from build123d import *

# Parameters (mm, degrees)
SKETCH1_R           = 1.6
SKETCH1_R_2         = 20
BOSS_EXTRUDE2_DEPTH = 1.7
BOSS_EXTRUDE3_START = -1.7
SKETCH2_R           = 1.5
BOSS_EXTRUDE3_DEPTH = 1.7
SKETCH3_W           = 67.365157796
SKETCH3_H           = 36
CUT_EXTRUDE1_DEPTH  = 1.7
FILLET1_R           = 3


with BuildPart() as part:
    # Sketch1 → Boss-Extrude2 (new body)
    with BuildSketch(Plane(origin=(0, 0, 0), x_dir=(1, 0, 0), z_dir=(0, 1, 0))):
        with BuildLine():
            Line((-17.673720383, -21.068687852), (-2.459890554, -40.906514899))
            ThreePointArc((-2.459890554, -40.906514899), (0, -42.12), (2.459890554, -40.906514899))
            Line((2.459890554, -40.906514899), (17.673720383, -21.068687852))
            ThreePointArc((17.673720383, -21.068687852), (19.445436483, -19.445436483), (21.068687852, -17.673720383))
            Line((21.068687852, -17.673720383), (40.906514899, -2.459890554))
            ThreePointArc((40.906514899, -2.459890554), (42.12, 0), (40.906514899, 2.459890554))
            Line((40.906514899, 2.459890554), (21.068687852, 17.673720383))
            ThreePointArc((21.068687852, 17.673720383), (19.445436483, 19.445436483), (17.673720383, 21.068687852))
            Line((17.673720383, 21.068687852), (2.459890554, 40.906514899))
            ThreePointArc((2.459890554, 40.906514899), (0, 42.12), (-2.459890554, 40.906514899))
            Line((-2.459890554, 40.906514899), (-17.673720383, 21.068687852))
            ThreePointArc((-17.673720383, 21.068687852), (-19.445436483, 19.445436483), (-21.068687852, 17.673720383))
            Line((-21.068687852, 17.673720383), (-40.906514899, 2.459890554))
            ThreePointArc((-40.906514899, 2.459890554), (-42.12, 0), (-40.906514899, -2.459890554))
            Line((-40.906514899, -2.459890554), (-21.068687852, -17.673720383))
            ThreePointArc((-21.068687852, -17.673720383), (-19.445436483, -19.445436483), (-17.673720383, -21.068687852))
        make_face()
        with Locations(Location((0, -39.02, 0), (0, 0, 270))):
            Circle(SKETCH1_R, mode=Mode.SUBTRACT)
        with Locations(Location((0, 0, 0), (0, 0, 270))):
            Circle(SKETCH1_R_2, mode=Mode.SUBTRACT)
        with Locations(Location((-39.02, 0, 0), (0, 0, 270))):
            Circle(SKETCH1_R, mode=Mode.SUBTRACT)
        with Locations(Location((39.02, 0, 0), (0, 0, 270))):
            Circle(SKETCH1_R, mode=Mode.SUBTRACT)
        with Locations(Location((0, 39.02, 0), (0, 0, 270))):
            Circle(SKETCH1_R, mode=Mode.SUBTRACT)
    extrude(amount=BOSS_EXTRUDE2_DEPTH)

    # Sketch2 → Boss-Extrude3 (add)
    with BuildSketch(Plane(origin=(0, 1.7, 0), x_dir=(1, 0, 0), z_dir=(0, 1, 0)).offset(BOSS_EXTRUDE3_START)):
        with BuildLine():
            Line((-30.78, -47.52), (-30.78, -10.226017059))
            Line((-30.78, -10.226017059), (-21.068687852, -17.673720383))
            ThreePointArc((-21.068687852, -17.673720383), (-19.445436483, -19.445436483), (-17.673720383, -21.068687852))
            Line((-17.673720383, -21.068687852), (-2.459890554, -40.906514899))
            ThreePointArc((-2.459890554, -40.906514899), (0, -42.12), (2.459890554, -40.906514899))
            ThreePointArc((2.459890554, -40.906514899), (-3.472049402, -45.77668656), (-10.946495328, -47.52))
            Line((-10.946495328, -47.52), (-30.78, -47.52))
        make_face()
        with Locations(Location((-9.5, -44.02, 0), (0, 0, 270))):
            Circle(SKETCH2_R, mode=Mode.SUBTRACT)
        with Locations(Location((-27.28, -44.02, 0), (0, 0, 270))):
            Circle(SKETCH2_R, mode=Mode.SUBTRACT)
        with Locations(Location((-27.28, -23.7, 0), (0, 0, 270))):
            Circle(SKETCH2_R, mode=Mode.SUBTRACT)
    extrude(amount=BOSS_EXTRUDE3_DEPTH)

    # Sketch3 → Cut-Extrude1 (cut)
    with BuildSketch(Plane(origin=(0, 1.7, 0), x_dir=(1, 0, 0), z_dir=(0, 1, 0))):
        with Locations((0, 26)):
            Rectangle(SKETCH3_W, SKETCH3_H)
    extrude(amount=-CUT_EXTRUDE1_DEPTH, mode=Mode.SUBTRACT)

    # Fillet1
    fillet1_edges = [part.edges().sort_by_distance(p)[0] for p in [
        (-18.33030278, 0.85, -8),
        (18.33030278, 0.85, -8),
        (-33.682578898, 0.85, -8),
        (33.682578898, 0.85, -8),
        (-30.78, 0.85, 47.52),
    ]]
    fillet(fillet1_edges, radius=FILLET1_R)


solid = part.part
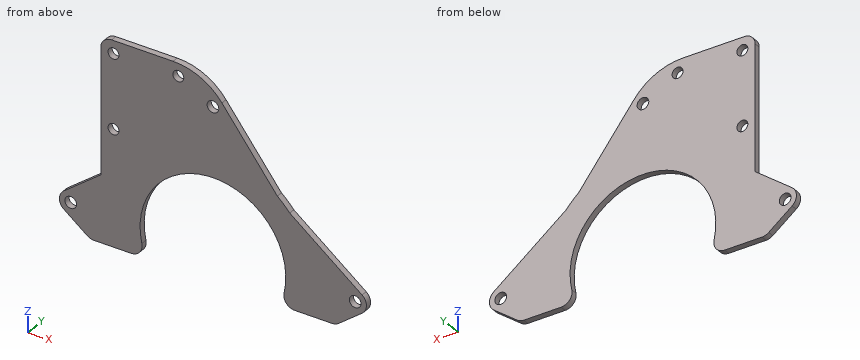
The listing builds one solid part. Answer for the finished solid, in the listing's coordinates (mm). Round coordinates to 2 decimals unless told otherwise and drop trailing zeros. Write each loop counter-clockwise with the first axis right and the second up, starting at its lowest first coordinate (ties: lowest second). Pieces come first, ordered by that corner, then holes. Notation, with made-up numbers: M 65,-35 L 109,-35 A9 cw 109,-27 Z; hole C 25.25,40.5 d8. An arc over 180 degrees is marked long. Write each question's results on one line, items separated by ' | '. Start each with the question number.
(1) Find the intervals of material crossed by line 1 (X direction, y = 1.35, z = -0.5); line 2 (X direction, y = 0.55, z = 44.02); line 3 (Z direction, x = -27, y = 0.4), in increasing order.
(2) This flat-tipped pin is pushed along its axis until it touches: P1, Ø1, axis at y = 0, z = 7.5, coming from the -X side. Where does it stop, or does it pass through?
(3) The part is cut by section A-A, the plane z = 0. Write down the section's boundary in (x, y), and give its area (3 significant figures).
(4) The part is cut by section D-D, the plane y = 1.15. Write down the section's boundary in (x, z), and give its area (3 significant figures).
(5) The part is cut by section B-B, the plane x = 0. Write down the section's boundary in (y, z), and give its area (3 significant figures).
(6) The part is cut by section C-C, the plane z = 14.5. Write down the section's boundary in (x, y), and give its area (3 significant figures).
Worked answers:
1) line 1: x = -42.08 to -40.54, -37.5 to -19.99, 19.99 to 37.5, 40.54 to 42.08 | line 2: x = -30.78 to -28.78, -25.78 to -11, -8 to -0.65 | line 3: z = -8 to 22.23, 25.17 to 42.55, 45.49 to 47.52
2) P1: stops at x = -34.99
3) outline: M -42.12,0 L -40.62,0 L -40.62,1.7 L -42.12,1.7 Z; M -37.42,0 L -20,0 L -20,1.7 L -37.42,1.7 Z; M 20,0 L 37.42,0 L 37.42,1.7 L 20,1.7 Z; M 40.62,0 L 42.12,0 L 42.12,1.7 L 40.62,1.7 Z | area: 64.3 mm²
4) outline: M -40.91,-2.46 L -34.49,-7.38 A3 ccw -32.66,-8 L -22.45,-8 A3 ccw -19.52,-4.35 A20 cw long 19.52,-4.35 A3 ccw 22.45,-8 L 32.66,-8 A3 ccw 34.49,-7.38 L 40.91,-2.46 A3.1 ccw 40.91,2.46 L 21.07,17.67 A27.5 ccw 17.67,21.07 L 2.46,40.91 A16.89 ccw -10.95,47.52 L -27.78,47.52 A3 ccw -30.78,44.52 L -30.78,10.23 L -40.91,2.46 A3.1 ccw Z; hole C -39.02,0 d3.2; hole C -27.28,23.7 d3; hole C -27.28,44.02 d3; hole C -9.5,44.02 d3; hole C 0,39.02 d3.2; hole C 39.02,0 d3.2 | area: 1,980 mm²
5) outline: M 0,20 L 1.7,20 L 1.7,37.42 L 0,37.42 Z; M 0,40.62 L 1.7,40.62 L 1.7,43.49 L 0,43.49 Z | area: 34.5 mm²
6) outline: M -30.78,0 L -13.77,0 L -13.77,1.7 L -30.78,1.7 Z; M 13.77,0 L 25.21,0 L 25.21,1.7 L 13.77,1.7 Z | area: 48.3 mm²
